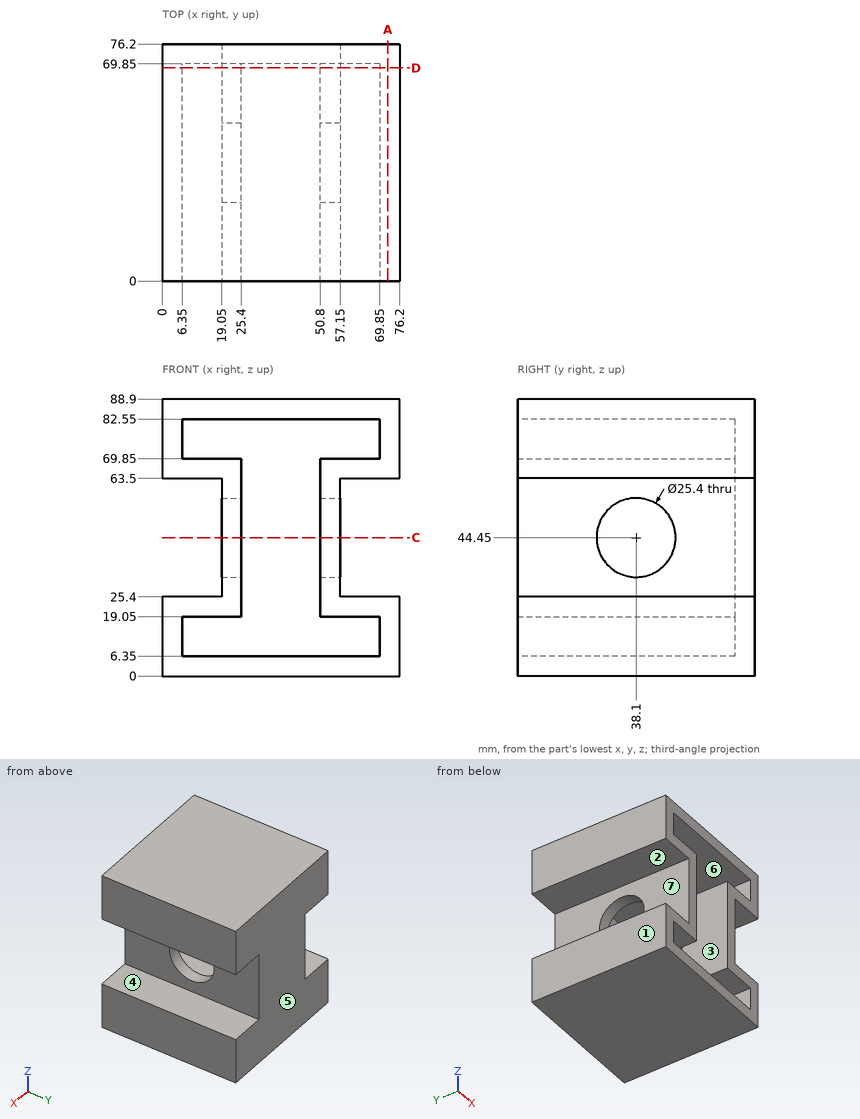
Design review of the part shown in the three views and the two pictorial views. Dimensions are in mm from the part's minimum x, y and z. A direction names the side the tool comes from. Give positions to 0.01 mm unless a question says otherwise; leave off trailing zeros. Loops run counter-clockwise (first coordinate to the right, second up) from the corner with the lowest first, then second, coordinate; pieces in that order, holes last. Notation, with made-up numbers: M 0.5,-34 L 46.5,-34 A22 ccw 46.5,-11 Z; hole C -32.5,75.5 d9. An arc over 180 degrees is marked long. Answer as a JSON object with one key per item and string values. Group by question number.
Q1. Add section C-C on z = 44.45. Give the boundary of the cut face in (x, y).
Q2. Add section D-D on y = 68.5. Give the boundary of the cut face in (x, z).
Q3. Insertion check: P1, Ø2, axis at y = 62.5, z = 37, coming from the -X side; P2, Ø2, axis at y = 22, z = 48.5, coming from the +X side; P3, Ø23, axis at y = 38.1, z = 44.45, coming from the -X side. Each pin has a flat end and moves straight along its axis. Give the tip position at first contact, or say it passes through.
Q4. Add section A-A on x = 72.5. Give the boundary of the cut face in (y, z).
Q5. Mouldability with a two-part tool opening along X and no side actions: class the marked faces 1, 2 and 3 as +X half, -X half, draft (parallel to the pull), parting line (faces both ways), or undercut.
Q6. For probe 1 along Z at (x, y) = (68.5, 59); probe 2 along Z at (x, y) = (23, 38.1); probe 3 along Y at (x, z) = (20, 44), list the stretches that pass through material, from the lowest coordinate up. Write a range as [from, to].
Q7. Tool access review of the marked faces 4, 5, 6 and 7: name each direction out of +Z, -Z, +X, -X, +Y, -Y from which nothing blocks a thin tool from reaching the whole face with its end or side.
Checked values:
{
 "1": {"outline": "M 19.05,0 L 25.4,0 L 25.4,25.4 L 19.05,25.4 Z; M 19.05,50.8 L 25.4,50.8 L 25.4,69.85 L 50.8,69.85 L 50.8,50.8 L 57.15,50.8 L 57.15,76.2 L 19.05,76.2 Z; M 50.8,0 L 57.15,0 L 57.15,25.4 L 50.8,25.4 Z"},
 "2": {"outline": "M 0,0 L 76.2,0 L 76.2,25.4 L 57.15,25.4 L 57.15,63.5 L 76.2,63.5 L 76.2,88.9 L 0,88.9 L 0,63.5 L 19.05,63.5 L 19.05,25.4 L 0,25.4 Z; hole M 6.35,6.35 L 69.85,6.35 L 69.85,19.05 L 50.8,19.05 L 50.8,69.85 L 69.85,69.85 L 69.85,82.55 L 6.35,82.55 L 6.35,69.85 L 25.4,69.85 L 25.4,19.05 L 6.35,19.05 Z"},
 "3": {"P1": "x = 19.05", "P2": "x = 57.15", "P3": "through"},
 "4": {"outline": "M 0,0 L 76.2,0 L 76.2,25.4 L 0,25.4 Z; M 0,63.5 L 76.2,63.5 L 76.2,88.9 L 0,88.9 Z"},
 "5": {"face 1": "-X half", "face 2": "draft", "face 3": "undercut"},
 "6": {"probe 1": "[0, 6.35], [19.05, 25.4], [63.5, 69.85], [82.55, 88.9]", "probe 2": "[0, 6.35], [19.05, 31.75], [57.15, 69.85], [82.55, 88.9]", "probe 3": "[0, 25.41], [50.79, 76.2]"},
 "7": {"face 4": "+X, +Y, -Y", "face 5": "+Z, -Z, +X, -X, +Y", "face 6": "-Y", "face 7": "-X, +Y, -Y"}
}
